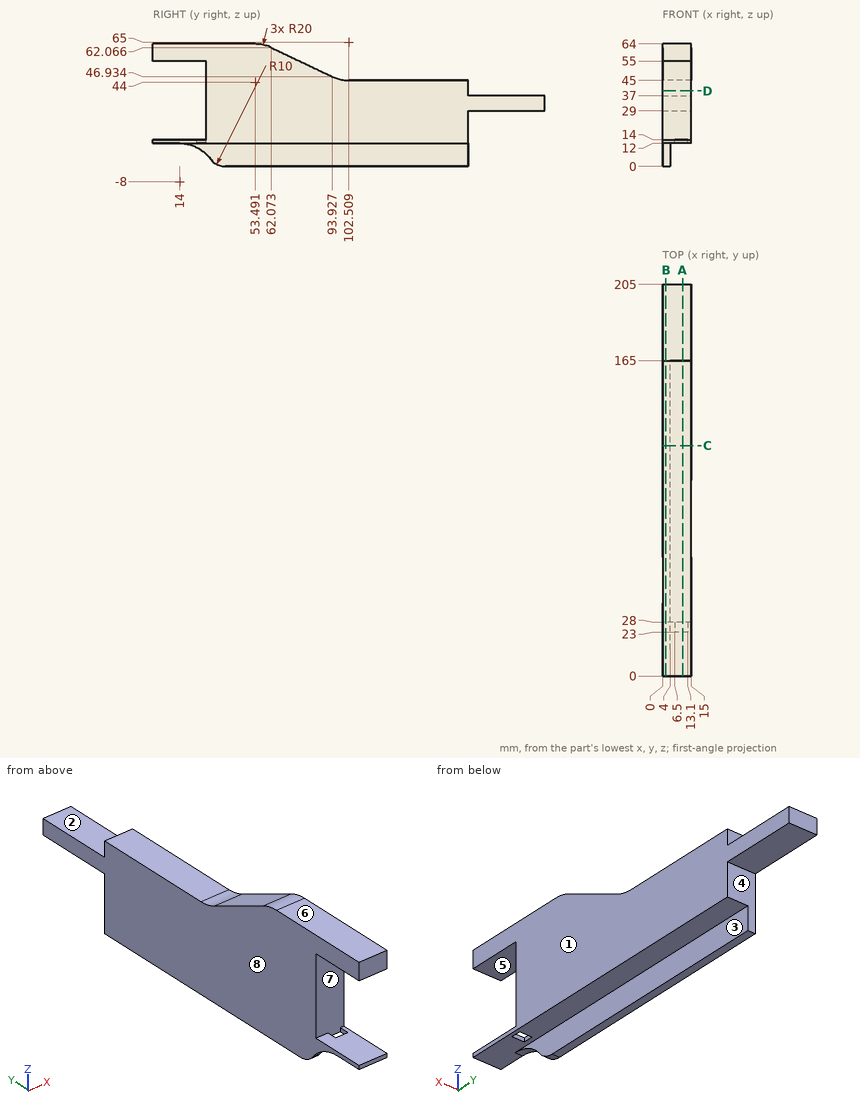
Could you check a few things on this drawing? It's one solid part, dimensions in mm from its lowest x, y, z. A direction names the side the tool comes from. Round coordinates to 2 decimals unless told otherwise and drop trailing zeros. Write each loop counter-clockwise with the first axis right and the second up, starting at its lowest first coordinate (ties: lowest second). Pieces come first, ordered by that corner, then holes. Notation, with made-up numbers: (18, 29.25) -> (59, 29.25) arc R22 cw to (59, 40.25) -> close; hole circle Ø6 at (68.5, 57). An arc over 180 degrees is marked (long way). Use one line per item in the form item = value. Start each with the question number.
Q1. Which directions (+Z, -Z, +X, -X, +Y, -Y) give clear straight access to the entire face, cutting with the end or side of a thin tool? Please do the marked faces 1, 2, 3, 4 and 5.
Q2. Imagine slicing it at A-A (x = 10.5). Please give me the cut outline in (y, z) (1 decimal), then the cut area to 3 significant figures.
Q3. Imagine slicing it at D-D (z = 39.5). Please give me the cut outline in (x, y).
Q4. Imagine slicing it at C-C (y = 120.5). Please give me the cut outline in (x, z), then the cut area to 3 significant figures.
Q5. I'm going to push flat-ended pins straight in: P1, Ø5, axis at x = 9.5, z = 40.5, coming from the +Y side; P2, Ø3, axis at x = 4, y = 120, coming from the +Z side; P3, Ø9, axis at x = 6, z = 41, coming from the +Y side; P4, Ø4.5, axis at x = 6, y = 190.5, coming from the +Z side. Where does each tip first touch, or does it pass through?
Q6. We'd pull the mould along Z, two halves only. Please class the marked faces 6, 7 and 8: +Z half, -Z half, draft (parallel to the pull), parting line (faces both ways), or undercut.
Q7. If I drill on probe 1 along Y at (x, z) = (10.5, 12.5); probe 2 along Y at (x, z) = (8.5, 21.5); probe 3 along Y at (x, z) = (3.75, 32), over which ranges is the centre line in solid material (lowest first)? Write a range as [from, to].
Q8. Imagine slicing it at B-B (x = 1.75). Please give me the cut outline in (y, z) (1 decimal), then the cut area to 3 significant figures.
Worked out:
q1.face_1 = +Z, -Z, +X, +Y, -Y
q1.face_2 = +Z, +X, -X, +Y
q1.face_3 = -Z, +X, +Y, -Y
q1.face_4 = -Z, +X, -X, +Y
q1.face_5 = +X, -X, -Y
q2.outline = (0, 12) -> (23, 12) -> (23, 14) -> (0, 14) -> close; (0, 55) -> (28, 55) -> (28, 12) -> (165, 12) -> (165, 29) -> (205, 29) -> (205, 37) -> (165, 37) -> (165, 45) -> (102.5, 45) arc R20 cw to (93.9, 46.9) -> (62.1, 62.1) arc R20 ccw to (53.5, 64) -> (0, 64) -> close
q2.area = 6,090 mm^2
q3.outline = (0, 28) -> (15, 28) -> (15, 165) -> (0, 165) -> close
q4.outline = (0, 0) -> (4, 0) -> (4, 12) -> (15, 12) -> (15, 45) -> (0, 45) -> close
q4.area = 543 mm^2
q5.P1 = 165
q5.P2 = 45
q5.P3 = 205
q5.P4 = 37
q6.face_6 = +Z half
q6.face_7 = undercut
q6.face_8 = draft
q7.probe_1 = [0, 23], [28, 165]
q7.probe_2 = [28, 165]
q7.probe_3 = [28, 205]
q8.outline = (0, 12) -> (14, 12) arc R20 cw to (30, 4) arc R10 ccw to (38, 0) -> (165, 0) -> (165, 29) -> (205, 29) -> (205, 37) -> (165, 37) -> (165, 45) -> (102.5, 45) arc R20 cw to (93.9, 46.9) -> (62.1, 62.1) arc R20 ccw to (53.5, 64) -> (0, 64) -> (0, 55) -> (28, 55) -> (28, 14) -> (0, 14) -> close
q8.area = 7,750 mm^2
